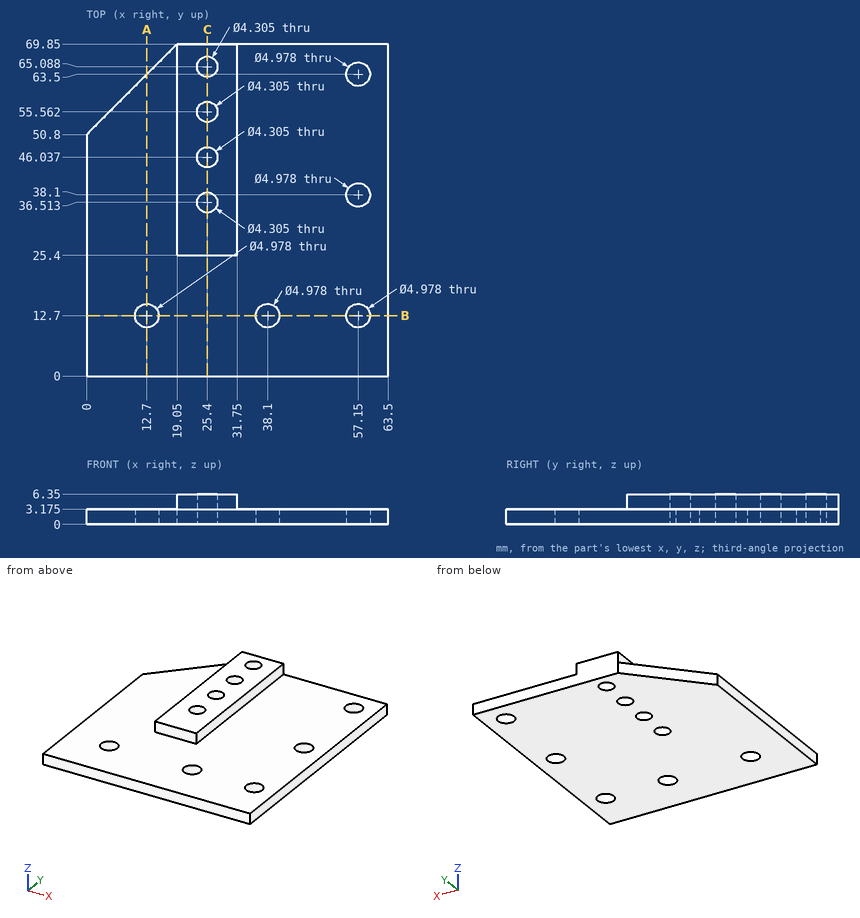
Here's the drawing with two shaded views (mm, measured from the low corner). I have some questions. Give positions to 0.01 mm unless a question says otherwise; leave off trailing zeros. Write each loop counter-clockwise with the first axis right and the second up, starting at its lowest first coordinate (ties: lowest second). Pieces come first, ordered by that corner, then holes. Notation, with made-up numbers: (67.5, -27) -> (74.5, -27) arc R29 ccw to (74.5, 3) -> close; hole circle Ø4 at (28, -15). An arc over 180 degrees is marked (long way). Use one line per item in the form item = value. Start each with the question number.
1. Imagine slicing it at C-C on x = 25.4. State how many separate pieces and enclosed holes the cut face has.
2. If I drill on L1, parallel to Y at x = 38.1, z = 2; L2, parallel to Z at x = 31, y = 7 (1 decimal); L3, parallel to Y at x = 12.7, z = 1.4, over which ranges is the centre line in solid material (lowest first)?
3. Imagine slicing it at A-A on x = 12.7. List the corners of the cut face in (y, z) for me (1 decimal), plus the area to 3 significant figures.
4. Will these pins go through, and if not, where does the flat tip stop? pin 1 Ø3 at (x, y) = (38.1, 12.7) entering from +Z; pin 2 Ø2 at (x, z) = (8, 1.5) entering from +Y; pin 3 Ø10 at (x, y) = (9.5, 61.5) entering from +Z (1 decimal); pin 4 Ø2 at (y, z) = (41, 4.5) entering from +X.
5. Imagine slicing it at B-B on y = 12.7. List the corners of the cut face in (x, z) for me (1 decimal), plus the area to 3 significant figures.
Entries:
q1.separate_pieces = 5
q1.enclosed_holes = 0
q2.L1 = 0 to 10.21, 15.19 to 69.85
q2.L2 = 0 to 3.2
q2.L3 = 0 to 10.21, 15.19 to 63.5
q3.outline = (0, 0) -> (10.2, 0) -> (10.2, 3.2) -> (0, 3.2) -> close; (15.2, 0) -> (63.5, 0) -> (63.5, 3.2) -> (15.2, 3.2) -> close
q3.area = 186 mm²
q4.pin_1 = through
q4.pin_2 = 59.8
q4.pin_3 = 3.2
q4.pin_4 = 31.75
q5.outline = (0, 0) -> (10.2, 0) -> (10.2, 3.2) -> (0, 3.2) -> close; (15.2, 0) -> (35.6, 0) -> (35.6, 3.2) -> (15.2, 3.2) -> close; (40.6, 0) -> (54.7, 0) -> (54.7, 3.2) -> (40.6, 3.2) -> close; (59.6, 0) -> (63.5, 0) -> (63.5, 3.2) -> (59.6, 3.2) -> close
q5.area = 154 mm²
